For this review, take the finished solid that the model builds, in its own axes (mm). Coordinates: 2 decimals unless noted, no trailing zeros. Loops run counter-clockwise (first coordinate to the right, second up) from the corner with the lowest first, then second, coordinate; pieces in that order, holes last.
1. Take a section at B-B, the plane x = 105. State the section outline as (y, z) points.
2. Take a section at A-A, the plane x = 200. State the section outline as (y, z) points, then the cut area to 3 significant figures.
3. To check wall thickness, follow probe 1 along Z at (x, y) = (200, 35); probe 2 along Y at (x, z) = (0, 23); probe 3 along Y at (x, z) = (129, 15). State the ranges of each line that lie inside material, in increasing order.
4. Take a section at C-C, the plane x = 0. State the section outline as (y, z) points.
5. Take a section at D-D, the plane y = 92. State the section outline as (x, z) points.
6. Clearance check with flat-ended pins moving along their axes: P1, Ø12, axis at x = 28, y = -5, coming from the -Z side; P2, Ø4, axis at x = 100, z = 19, coming from the +Y side; P3, Ø5, axis at y = -53, z = 26.5, coming from the +X side. State where each tip first meets the part, or that it passes through.
```python
from build123d import *

# Parameters (mm, degrees)
F0_R          = 14.5
F0_R_2        = 13.5
F1_DEPTH      = 30
F3_DEPTH      = 200
F4_END_RADIUS = 13.5
F3_FACE_R     = 10
F3_FACE_R_2   = 9
F4_REACH      = 228.2852713475
F6_DEPTH      = 150
F8_END_RADIUS = 13.5
F3_FACE1_R    = 10
F3_FACE1_R_2  = 9
F8_REACH      = 242.7852713475


with BuildPart() as f1:
    # F0 (on Top) → F1 (new body)
    with BuildSketch(Plane.XY):
        Circle(F0_R)
        Circle(F0_R_2, mode=Mode.SUBTRACT)
    extrude(amount=F1_DEPTH)

    # F2 (on Right) → F3 (join)
    with BuildSketch(Plane.YZ):
        with BuildLine():
            ThreePointArc((10, 15), (-7.0710678119, 22.0710678119), (0, 5))
            ThreePointArc((0, 5), (7.0710678119, 7.9289321881), (10, 15))
        make_face()
        with BuildLine():
            ThreePointArc((9, 15), (6.3639610307, 8.6360389693), (0, 6))
            ThreePointArc((0, 6), (-6.3639610307, 21.3639610307), (9, 15))
        make_face(mode=Mode.SUBTRACT)
    extrude(amount=F3_DEPTH)

    f4_end = (Plane(origin=(0, 0, 15), x_dir=(-1, 0, 0), z_dir=(0, 0, -1)) * Cylinder(F4_END_RADIUS, 893.6117311859, mode=Mode.PRIVATE)).faces().sort_by_distance((-13.5, 0, 15))[0]
    # F3_face (on face) → F4 (cut, up to the whole of a round face its end follows)
    with BuildSketch(Plane(origin=(0, 0, 15), x_dir=(0, 1, 0), z_dir=(-1, 0, 0))):
        Circle(F3_FACE_R)
        Circle(F3_FACE_R_2, mode=Mode.SUBTRACT)
    f4_long = extrude(amount=-F4_REACH, mode=Mode.PRIVATE)
    add(split(f4_long, bisect_by=f4_end, keep=Keep.BOTTOM, mode=Mode.PRIVATE), mode=Mode.SUBTRACT)

    # F5 (on Front) → F6 (join)
    with BuildSketch(Plane.XZ):
        with BuildLine():
            ThreePointArc((214.5, 15), (200, 29.5), (185.5, 15))
            ThreePointArc((185.5, 15), (200, 0.5), (214.5, 15))
        make_face()
        with BuildLine():
            ThreePointArc((213.5, 15), (200, 1.5), (186.5, 15))
            ThreePointArc((186.5, 15), (200, 28.5), (213.5, 15))
        make_face(mode=Mode.SUBTRACT)
    extrude(amount=F6_DEPTH)

    # F7: F1 across plane


with BuildPart() as f1_1:
    add(f1.part)
    add(f1.part.mirror(Plane.XZ))

    f8_end = (Plane(origin=(200, 0, 15), x_dir=(0, 0, 1), z_dir=(0, 1, 0)) * Cylinder(F8_END_RADIUS, 1242.7785728256, mode=Mode.PRIVATE)).faces().sort_by_distance((186.5, -146.9757976235, 15))[0]
    # F3_face1 (on face) → F8 (cut, up to the whole of a round face its end follows)
    with BuildSketch(Plane(origin=(200, 0, 15), x_dir=(0, 1, 0), z_dir=(1, 0, 0))):
        Circle(F3_FACE1_R)
        Circle(F3_FACE1_R_2, mode=Mode.SUBTRACT)
    f8_long = extrude(amount=-F8_REACH, mode=Mode.PRIVATE)
    add(split(f8_long, bisect_by=f8_end, keep=Keep.BOTTOM, mode=Mode.PRIVATE), mode=Mode.SUBTRACT)


solid = f1_1.part
```
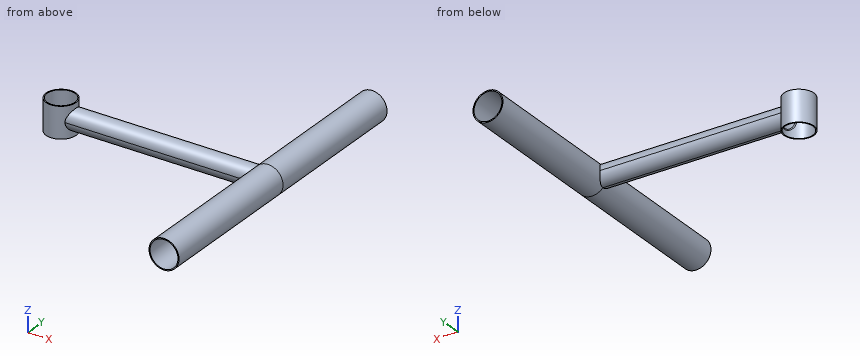
Results list:
1. outline: circle Ø20 at (0, 15); hole circle Ø18 at (0, 15)
2. outline: (-150, 0.5) - (150, 0.5) - (150, 1.5) - (-150, 1.5) - close; (-150, 28.5) - (150, 28.5) - (150, 29.5) - (-150, 29.5) - close
2. area: 600 mm2
3. probe 1: z = 0.5 to 1.5, 28.5 to 29.5
3. probe 2: y = -14.5 to -13.5, 13.5 to 14.5
3. probe 3: y = -10 to -9, 9 to 10
4. outline: (-14.5, 0) - (-13.5, 0) - (-13.5, 30) - (-14.5, 30) - close; (13.5, 0) - (14.5, 0) - (14.5, 30) - (13.5, 30) - close
5. outline: circle Ø29 at (200, 15); hole circle Ø27 at (200, 15)
6. P1: stops at z = 5
6. P2: stops at y = 9.8
6. P3: stops at x = 211.37
